Geometry: final body of the model. Coordinates: model frame, mm. A direction names the side the tool comes from. Coordinates: 2 decimals unless noted, no trailing zeros. Write each loop counter-clockwise with the first axis right and the second up, starting at its lowest first coordinate (ties: lowest second). Pieces come first, ordered by that corner, then holes. Notation, with made-up numbers: (25, -24.5) -> (84, -24.5) arc R18 ccw to (84, -4.5) -> close; hole circle Ø5 at (57, 1.5). An arc over 180 degrees is marked (long way). One line per item, written item: value. Start each with the question number.
Autodesk Fusion 360 part; units mm, degrees
sketch "Boceto1" plane through (0, 0, 0) normal (0, 0, 1) x (1, 0, 0)
  circle A0 centre (0, 0) radius 12.5
  line L0 (12.5, 0) -> (-12.5, 0) construction
  circle A1 centre (0, 0) radius 4 construction
  circle A2 centre (0, 0) radius 2 construction
  circle A3 centre (7.5, 0) radius 1.5
  circle A4 centre (-7.5, 0) radius 1.5
  line L1 (7.5, -3.1754) -> (10.25, -1.5877)
  line L2 (10.25, -1.5877) -> (10.25, 1.5877)
  line L3 (10.25, 1.5877) -> (7.5, 3.1754)
  line L4 (7.5, 3.1754) -> (4.75, 1.5877)
  line L5 (4.75, 1.5877) -> (4.75, -1.5877)
  line L6 (4.75, -1.5877) -> (7.5, -3.1754)
  line L7 (-7.5, -3.1754) -> (-4.75, -1.5877)
  line L8 (-4.75, -1.5877) -> (-4.75, 1.5877)
  line L9 (-4.75, 1.5877) -> (-7.5, 3.1754)
  line L10 (-7.5, 3.1754) -> (-10.25, 1.5877)
  line L11 (-10.25, 1.5877) -> (-10.25, -1.5877)
  line L12 (-10.25, -1.5877) -> (-7.5, -3.1754)
  point P0 (7.5, 0)
  point P1 (-7.5, 0)
  dimension "d1" = 25
  dimension "d9" = 8
  dimension "d10" = 4
  dimension "d11" = 3
  dimension "d12" = 3
  dimension "d13" = 2.75
  dimension "d14" = 2.75
  dimension "d29" = 7.5
  dimension "d30" = 7.5
extrude "Extruir1" add sketch "Boceto1" against normal blind 10 contours A0 | A3 | A4 | L1 L2 L3 L4 L5 L6 | L7 L8 L9 L10 L11 L12
ref_plane "PlanoDeObra1" through (0, 0, 10) normal (0, 0, 1) x (1, 0, 0)
sketch "Boceto2" plane through (0, 0, 10) normal (0, 0, 1) x (1, 0, 0)
  circle A0 centre (0, 0) radius 12.5
  circle A1 centre (0, 0) radius 4
  dimension "d5" = -8.5
loft "Solevación1" add profiles "Boceto2" section 1 contours A1 section 2 face at (-3.3879, -0.621, 0)
sketch "Boceto3" plane through (0, 0, 10) normal (0, 0, 1) x (-1, 0, 0)
  circle A0 centre (0, 0) radius 4
  circle A1 centre (0, 0) radius 2
  dimension "d6" = 4
extrude "Extruir2" cut sketch "Boceto3" along normal mid plane 78 contours A1
sketch "Boceto4" plane through (0, 0, 10) normal (0, 0, 1) x (-1, 0, 0)
  circle A0 centre (0, 0) radius 2
  circle A1 centre (0, 0) radius 4
extrude "Extruir5" cut sketch "Boceto1" along normal blind 14 contours L1 L2 L3 L4 L5 L6
extrude "Extruir6" cut sketch "Boceto1" along normal blind 29 contours A3
extrude "Extruir7" cut sketch "Boceto1" along normal mid plane 60 contours A3
extrude "Extruir8" cut sketch "Boceto1" along normal blind 25 contours L7 L8 L9 L10 L11 L12
extrude "Extruir9" cut sketch "Boceto1" along normal mid plane 52 contours A4
Q1. Cut plane B-B on z = 5.5. Output: boundary loops of the cut face in (x, y) (3 decimals), and give its area (3 significant figures).
Q2. Line query: L1, parallel to X at y = -0.5, z = -5.5; L2, parallel to X at y = 0, z = 2.25; L3, parallel to Y at x = 7.5, z = -3. Output: solid intervals per line, ascending. Write a range as from..to.
Q3. Cut plane C-C on y = 0. Count the separate pieces of the cut face and the enclosed holes in it, and give its area (3 significant figures).
Q4. Cut plane A-A on x = 0. Output: boundary loops of the cut face in (y, z), and give its area (3 significant figures).
Q5. Draft query along X for faces 1 (the flat face through (-8.894, -2.37, 1.957)), 2 (the flat face through (0, -3, -10)), 3 (the cylindrical face through (11.923, 3.755, -4.93)). Return one class per face: pulls with the +X half, pulls with the -X half, needs draft (parallel to the pull), parting line crosses it, or undercut.
Q6. First-contact query: P1, Ø1.3, axis at y = 0.5, z = 1.5, coming from the -X side; P2, Ø1.6, axis at y = -1, z = 6.5, coming from the -X side; P3, Ø3, axis at x = 1.5, z = 3.5, coming from the +Y side. Flat tips, straight axial feed; report the tip coordinate or a pass-through.
Q7. Access query for faces 4 (the flat face through (-4.75, 0, 4)), 5 (the cylindrical face through (-9, 0, -5)). Directions: +Z, -Z, +X, -X, +Y, -Y. A direction counts if a zero-diameter tool reaches every point of the face in a straight line with its end or side. Return the directions, or none.
Q8. Cut plane D-D on z = -7. Output: boundary loops of the cut face in (x, y), and give its area (3 significant figures).
Solution:
1. outline: (-7.221, -3.014) arc R7.825 ccw to (7.221, -3.014) -> (4.75, -1.588) -> (4.75, 1.588) -> (7.221, 3.014) arc R7.825 ccw to (-7.221, 3.014) -> (-4.75, 1.588) -> (-4.75, -1.588) -> close; hole circle Ø4 at (0, 0)
1. area: 152 mm²
2. L1: -12.49..-8.91, -6.09..-1.94, 1.94..6.09, 8.91..12.49
2. L2: -10.59..-10.25, -4.75..-2, 2..4.75, 10.25..10.59
2. L3: -10..-1.5, 1.5..10
3. separate pieces: 4
3. enclosed holes: 0
3. area: 210 mm²
4. outline: (-12.5, -10) -> (-2, -10) -> (-2, 10) -> (-4, 10) -> (-12.5, 0) -> close; (2, -10) -> (12.5, -10) -> (12.5, 0) -> (4, 10) -> (2, 10) -> close
4. area: 335 mm²
5. face 1: undercut
5. face 2: needs draft
5. face 3: parting line crosses it
6. P1: x = -11.77
6. P2: x = -5.12
6. P3: y = 10.71
7. face 4: +Z
7. face 5: +Z, -Z
8. outline: circle Ø25 at (0, 0); hole circle Ø3 at (-7.5, 0); hole circle Ø4 at (0, 0); hole circle Ø3 at (7.5, 0)
8. area: 464 mm²
